Part model, mm, in its own coordinate system. A direction names the side the tool comes from. Round coordinates to 2 decimals unless told otherwise and drop trailing zeros. Loops run counter-clockwise (first coordinate to the right, second up) from the corner with the lowest first, then second, coordinate; pieces in that order, holes last.
1) Band-saw the part on A-A, the plane y = 24.65. Write the cut outline in (x, z), then the cut area to 3 significant figures.
2) Drop flat-ended pins along their axis: P1, Ø3, axis at y = 23, z = 3, coming from the +X side; P2, Ø2.5, axis at x = 11, z = 2.5, coming from the +Y side; P3, Ø3, axis at y = 22.5, z = 3.5, coming from the -X side. Give the stop position or say it passes through.
3) Band-saw the part on B-B, the plane x = -6. Write the cut outline in (y, z).
4) Band-saw the part on C-C, the plane z = 2.75. State how many separate pieces and enclosed holes the cut face has, then the cut area to 3 significant figures.
5) Mould opens along Y. For faces 1 (the flat face through (0, -8.35, 3)), 2 (the flat face through (0, 0, 6.35)), 3 (the cylindrical face through (6.43, -12, 3.13)) say: +Y half, -Y half, draft (parallel to the pull), parting line (faces both ways), or undercut.
6) 3-axis set-ups, long thin cutter, end or side, ignore diameter. For faces 4 (the flat face through (-12, -10.5, 3)), 5 (the flat face through (-23, 5, 3)), 6 (the flat face through (0, -0.35, 3)): which of +Z, -Z, +X, -X, +Y, -Y reach the whole face in a straight line?
7) Probe line 1 (X direction, y = -10, z = 6) (3 decimals); line 2 (Y direction, x = 21, z = 4.75); line 3 (Y direction, x = 23, z = 4). List the from-to ranges inside material, lowest first.
from build123d import *

# Parameters (mm, degrees)
F0_W      = 27.25
F0_H      = 21
F1_DEPTH  = 6.35
F2_R      = 0.4
F3_DEPTH  = 25.4
F5_DEPTH  = 6.35
F6_R      = 1.6
F7_DEPTH  = 25.4
F8_R      = 5
F9_R      = 2.5
F10_R     = 0.49999
F12_DEPTH = 25.4


# Not quite as in the source:
# - a fillet or chamfer is up to 0.001 mm smaller than in the source, because OpenCascade refuses the exact size


with BuildPart() as f1:
    # F0 (on Top) → F1 (new body)
    with BuildSketch(Plane.XY):
        Rectangle(F0_W, F0_H)
    extrude(amount=F1_DEPTH)

    # F2 (on face) → F3 (cut)
    with BuildSketch(Plane.XY.offset(6.35)):
        with Locations((11, 1)):
            Circle(F2_R)
        with Locations((11, 3)):
            Circle(F2_R)
        with Locations((11, 5)):
            Circle(F2_R)
        with Locations((11, 7)):
            Circle(F2_R)
        with Locations((11, 9)):
            Circle(F2_R)
        with Locations((11, -1)):
            Circle(F2_R)
        with Locations((11, -3)):
            Circle(F2_R)
        with Locations((11, -5)):
            Circle(F2_R)
        with Locations((11, -7)):
            Circle(F2_R)
        with Locations((11, -9)):
            Circle(F2_R)
        with Locations((-11, 9)):
            Circle(F2_R)
        with Locations((-11, 7)):
            Circle(F2_R)
        with Locations((-11, 5)):
            Circle(F2_R)
        with Locations((-11, 3)):
            Circle(F2_R)
        with Locations((-11, 1)):
            Circle(F2_R)
        with Locations((-11, -1)):
            Circle(F2_R)
        with Locations((-11, -3)):
            Circle(F2_R)
        with Locations((-11, -5)):
            Circle(F2_R)
        with Locations((-11, -7)):
            Circle(F2_R)
        with Locations((-11, -9)):
            Circle(F2_R)
    extrude(amount=-F3_DEPTH, mode=Mode.SUBTRACT)

    # F4 (on face) → F5 (join)
    with BuildSketch(Plane.XY.offset(6.35)):
        Polygon((5, 29), (0, 29), (-5, 29), (-5, 10.5), (0, 10.5), (5, 10.5), align=None)
        Polygon((-5, -10.5), (-5, -29), (0, -29), (5, -29), (5, -10.5), (0, -10.5), align=None)
        Polygon((-30, 5), (-30, 0), (-30, -5), (-13.625, -5), (-13.625, 0), (-13.625, 5), align=None)
        Polygon((30, 5), (13.625, 5), (13.625, 0), (13.625, -5), (30, -5), (30, 0), align=None)
    extrude(amount=-F5_DEPTH)

    # F6 (on face) → F7 (cut)
    with BuildSketch(Plane.XY.offset(6.35)):
        with Locations((-25.625, 0)):
            Circle(F6_R)
        with Locations((22.375, 0)):
            Circle(F6_R)
        with Locations((0, 24.65)):
            Circle(F6_R)
    extrude(amount=-F7_DEPTH, mode=Mode.SUBTRACT)

    # F8
    f8_edges = [f1.edges().sort_by_distance(p)[0] for p in [
        (-5, 10.5, 3.175),
        (-13.625, 5, 3.175),
        (-13.625, -5, 3.175),
        (-5, -10.5, 3.175),
        (5, 10.5, 3.175),
        (13.625, 5, 3.175),
        (13.625, -5, 3.175),
        (5, -10.5, 3.175),
    ]]
    fillet(f8_edges, radius=F8_R)

    # F9
    f9_edges = [f1.edges().sort_by_distance(p)[0] for p in [
        (-30, 5, 3.175),
        (-5, 29, 3.175),
        (5, 29, 3.175),
        (-30, -5, 3.175),
        (-5, -29, 3.175),
        (5, -29, 3.175),
        (30, 5, 3.175),
        (30, -5, 3.175),
    ]]
    fillet(f9_edges, radius=F9_R)

    # F10 (radius 0.5 in the source; OpenCascade refuses exactly that, so slightly less here)
    f10_edges = [f1.edges().sort_by_distance(p)[0] for p in [
        (-13.625, -10.5, 3.175),
        (13.625, -10.5, 3.175),
        (-13.625, 10.5, 3.175),
        (13.625, 10.5, 3.175),
    ]]
    fillet(f10_edges, radius=F10_R)

    # F11 (on face) → F12 (cut)
    with BuildSketch(Plane.XY.offset(6.35)):
        with BuildLine():
            Line((7, -0.35), (-7, -0.35))
            ThreePointArc((-7, -0.35), (-7.7071067812, -0.6428932188), (-8, -1.35))
            Line((-8, -1.35), (-8, -7.35))
            ThreePointArc((-8, -7.35), (-7.7071067812, -8.0571067812), (-7, -8.35))
            Line((-7, -8.35), (7, -8.35))
            ThreePointArc((7, -8.35), (7.7071067812, -8.0571067812), (8, -7.35))
            Line((8, -7.35), (8, -1.35))
            ThreePointArc((8, -1.35), (7.7071067812, -0.6428932188), (7, -0.35))
        make_face()
    extrude(amount=-F12_DEPTH, mode=Mode.SUBTRACT)


solid = f1.part
Reported:
1. outline: (-5, 0) - (-1.6, 0) - (-1.6, 6.35) - (-5, 6.35) - close; (1.6, 0) - (5, 0) - (5, 6.35) - (1.6, 6.35) - close
1. area: 43.2 mm2
2. P1: stops at x = 5
2. P2: stops at y = 10.51
2. P3: stops at x = -5
3. outline: (-12.5, 0) - (-8.35, 0) - (-8.35, 6.35) - (-12.5, 6.35) - close; (-0.35, 0) - (12.5, 0) - (12.5, 6.35) - (-0.35, 6.35) - close
4. separate pieces: 1
4. enclosed holes: 24
4. area: 1,140 mm2
5. face 1: undercut
5. face 2: draft
5. face 3: -Y half
6. face 4: +Z, -Z, -X, -Y
6. face 5: +Z, -Z, -X, +Y
6. face 6: +Z, -Z
7. line 1: x = -13.625 to 13.625
7. line 2: y = -5 to -0.82, 0.82 to 5
7. line 3: y = -5 to -1.47, 1.47 to 5
